CAD build for the part. Positions are in the model's coordinates, mm. Face numbers are marked on the shaded views. Give positions to 0.01 mm unless a question says otherwise; leave off trailing zeros. Order: outer loops, then holes, each group sorted by start corner. A loop starts at its lowest first (then second) coordinate and runs counter-clockwise, first axis right, second up. Notation, with made-up numbers: (85.25, -12) -> (115.25, -12) arc R21 ccw to (115.25, 25) -> close; hole circle Ø4 at (-10, 48.5). An arc over 180 degrees is marked (long way). Answer as CSV lines item,"result".
```python
from build123d import *

# Parameters (mm, degrees)
SKETCH_1_W           = 4.9
SKETCH_1_H           = 5.8
EXTRUDE_1_DEPTH      = 0.95
FILLET_1_R           = 0.2
CHAMFER_1_SIZE       = 0.2
EXTRUDE_2_DEPTH      = 0.05
EXTRUDE_2_DEPTH_BACK = 0.05
SKETCH_2_W           = 0.41
SKETCH_2_H           = 0.61
CHAMFER_2_SIZE       = 0.05
EXTRUDE_3_DEPTH      = 0.05
EXTRUDE_3_DEPTH_BACK = 0.05
SKETCH_3_W           = 4.15
SKETCH_3_H           = 3.85
SKETCH_3_W_2         = 0.41
SKETCH_3_H_2         = 0.15
SKETCH_3_W_3         = 0.375
SKETCH_3_H_3         = 0.41
SKETCH_3_W_4         = 0.15
CHAMFER_3_SIZE       = 0.05
SKETCH_4_R           = 0.15
CUT_EXTRUDE_1_DEPTH  = 0.01


with BuildPart() as part:
    # Эскиз1 → Бобышка-Вытянуть1 (new body)
    with BuildSketch(Plane(origin=(0, 0, 0), x_dir=(1, 0, 0), z_dir=(0, 1, 0))):
        Rectangle(SKETCH_1_W, SKETCH_1_H)
    extrude(amount=EXTRUDE_1_DEPTH)

    # Скругление1
    fillet_1_edges = [part.edges().sort_by_distance(p)[0] for p in [
        (2.45, 0.475, 2.9),
        (-2.45, 0.475, 2.9),
        (-2.45, 0.475, -2.9),
        (2.45, 0.475, -2.9),
    ]]
    fillet(fillet_1_edges, radius=FILLET_1_R)

    # Фаска1
    chamfer_1_edges = [part.edges().sort_by_distance(p)[0] for p in [
        (-2.45, 0.95, 0),
        (0, 0.95, -2.9),
        (2.45, 0.95, 0),
        (0, 0.95, 2.9),
        (2.391421356, 0.95, 2.841421356),
        (-2.391421356, 0.95, 2.841421356),
        (2.391421356, 0.95, -2.841421356),
        (-2.391421356, 0.95, -2.841421356),
    ]]
    chamfer(chamfer_1_edges, length=CHAMFER_1_SIZE)

    # Эскиз2 → Бобышка-Вытянуть2 (add, two sides: drawn at the far end of the back side and taken through both)
    with BuildSketch(Plane.XZ.offset(-EXTRUDE_2_DEPTH_BACK)):
        with Locations((0.635, -2.745)):
            Rectangle(SKETCH_2_W, SKETCH_2_H)
        with Locations((1.905, -2.745)):
            Rectangle(SKETCH_2_W, SKETCH_2_H)
        with Locations((-0.635, -2.745)):
            Rectangle(SKETCH_2_W, SKETCH_2_H)
        with Locations((-1.905, -2.745)):
            Rectangle(SKETCH_2_W, SKETCH_2_H)
    extrude(amount=EXTRUDE_2_DEPTH + EXTRUDE_2_DEPTH_BACK)

    # Фаска2
    chamfer_2_edges = [part.edges().sort_by_distance(p)[0] for p in [
        (-2.11, 0, -3.05),
        (-1.7, 0, -3.05),
        (1.7, 0, -3.05),
        (2.11, 0, -3.05),
        (0.43, 0, -3.05),
        (0.84, 0, -3.05),
        (-0.84, 0, -3.05),
        (-0.43, 0, -3.05),
    ]]
    chamfer(chamfer_2_edges, length=CHAMFER_2_SIZE)

    # Эскиз3 → Бобышка-Вытянуть3 (add, two sides: drawn at the far end of the back side and taken through both)
    with BuildSketch(Plane.XZ.offset(-EXTRUDE_3_DEPTH_BACK)):
        with Locations((0, 0.685)):
            Rectangle(SKETCH_3_W, SKETCH_3_H)
        with Locations((1.905, 2.975)):
            Rectangle(SKETCH_3_W_2, SKETCH_3_H_2)
        Polygon((1.7, 2.61), (2.075, 2.61), (2.11, 2.61), (2.11, 2.9), (1.7, 2.9), align=None)
        with Locations((-1.905, 2.975)):
            Rectangle(SKETCH_3_W_2, SKETCH_3_H_2)
        Polygon((-2.11, 2.61), (-2.075, 2.61), (-1.7, 2.61), (-1.7, 2.9), (-2.11, 2.9), align=None)
        with Locations((2.2625, -0.5)):
            Rectangle(SKETCH_3_W_3, SKETCH_3_H_3)
        with Locations((2.525, -0.5)):
            Rectangle(SKETCH_3_W_4, SKETCH_3_H_3)
        with Locations((-2.2625, -0.5)):
            Rectangle(SKETCH_3_W_3, SKETCH_3_H_3)
        with Locations((-2.525, -0.5)):
            Rectangle(SKETCH_3_W_4, SKETCH_3_H_3)
    extrude(amount=EXTRUDE_3_DEPTH + EXTRUDE_3_DEPTH_BACK)

    # Фаска3
    # the kernel refuses this chamfer: 0.05 mm, written as the material it adds along each edge
    with BuildSketch(Plane(origin=(-1.7, -0.05, 2.61), x_dir=(-0.02749587661058742, 0, 0.9996219169112966), z_dir=(0, 1, 0)), Plane(origin=(1.7, -0.05, 2.61), x_dir=(-0.9996219169112966, 0, -0.02749587661058718), z_dir=(0, 1, 0))) as chamfer_3_piece_1:
        Polygon((CHAMFER_3_SIZE * 0.999621916911, CHAMFER_3_SIZE * 0.0274958766106), (-CHAMFER_3_SIZE * 0.0274958766106, CHAMFER_3_SIZE * 0.999621916911), (0, 0), align=None)
    extrude(amount=0.178584149)
    # the kernel refuses this chamfer: 0.05 mm, written as the material it takes off along each edge
    with BuildSketch(Plane(origin=(-2.6, -0.178584149, -0.295), x_dir=(0.9996219169112966, 0, 0.02749587661058634), z_dir=(0, 1, 0)), Plane(origin=(2.6, -0.178584149, -0.705), x_dir=(-0.9996219169112965, 0, -0.027495876610591732), z_dir=(0, 1, 0)), Plane(origin=(2.6, -0.178584149, -0.295), x_dir=(0.02749587661058736, 0, -0.9996219169112966), z_dir=(0, 1, 0))) as chamfer_3_2_piece_1:
        Polygon((CHAMFER_3_SIZE * 0.999621916911, CHAMFER_3_SIZE * 0.0274958766106), (-CHAMFER_3_SIZE * 0.0274958766106, CHAMFER_3_SIZE * 0.999621916911), (0, 0), align=None)
    extrude(amount=0.357168299, mode=Mode.SUBTRACT)
    with BuildSketch(Plane(origin=(-2.11, -0.178584149, 2.61), x_dir=(-0.02749587661058742, 0, 0.9996219169112966), z_dir=(0, 1, 0))) as chamfer_3_2_piece_2_section:
        Polygon((CHAMFER_3_SIZE * 0.999621916911, CHAMFER_3_SIZE * 0.0274958766106), (-CHAMFER_3_SIZE * 0.0274958766106, CHAMFER_3_SIZE * 0.999621916911), (0, 0), align=None)
    chamfer_3_2_piece_2 = extrude(amount=0.178584149, mode=Mode.PRIVATE)
    chamfer_3_2_piece_2 = split(chamfer_3_2_piece_2, bisect_by=Plane(origin=(-2.075, -0.025, 2.627820513), z_dir=(-1, 0, 0)), keep=Keep.TOP, mode=Mode.PRIVATE)
    add(chamfer_3_2_piece_2, mode=Mode.SUBTRACT)
    with BuildSketch(Plane(origin=(-1.7, -0.178584149, 3.05), x_dir=(-0.9996219169112966, 0, 0.027495876610587302), z_dir=(0, 1, 0)), Plane(origin=(2.11, -0.178584149, 3.05), x_dir=(-0.9996219169112966, 0, 0.02749587661058742), z_dir=(0, 1, 0)), Plane(origin=(-2.6, -0.178584149, -0.705), x_dir=(0.9996219169112966, 0, -0.02749587661058742), z_dir=(0, 1, 0)), Plane(origin=(-2.11, -0.178584149, 3.05), x_dir=(-0.02749587661058742, 0, -0.9996219169112966), z_dir=(0, 1, 0)), Plane(origin=(1.7, -0.178584149, 3.05), x_dir=(-0.027495876610591732, 0, -0.9996219169112965), z_dir=(0, 1, 0))) as chamfer_3_2_piece_3:
        Polygon((CHAMFER_3_SIZE * 0.999621916911, -CHAMFER_3_SIZE * 0.0274958766106), (-CHAMFER_3_SIZE * 0.0274958766106, -CHAMFER_3_SIZE * 0.999621916911), (0, 0), align=None)
    extrude(amount=0.357168299, mode=Mode.SUBTRACT)
    with BuildSketch(Plane(origin=(2.11, -0.178584149, 2.61), x_dir=(0.02749587661058742, 0, 0.9996219169112966), z_dir=(0, 1, 0))) as chamfer_3_2_piece_4_section:
        Polygon((CHAMFER_3_SIZE * 0.999621916911, -CHAMFER_3_SIZE * 0.0274958766106), (-CHAMFER_3_SIZE * 0.0274958766106, -CHAMFER_3_SIZE * 0.999621916911), (0, 0), align=None)
    chamfer_3_2_piece_4 = extrude(amount=0.178584149, mode=Mode.PRIVATE)
    chamfer_3_2_piece_4 = split(chamfer_3_2_piece_4, bisect_by=Plane(origin=(2.075, -0.025, 2.627820513), z_dir=(1, 0, 0)), keep=Keep.TOP, mode=Mode.PRIVATE)
    add(chamfer_3_2_piece_4, mode=Mode.SUBTRACT)

    # Эскиз4 → Вырез-Вытянуть1 (cut)
    with BuildSketch(Plane(origin=(0, 0.95, 0), x_dir=(1, 0, 0), z_dir=(0, 1, 0))):
        with Locations(Location((1.85, 2.3, 0), (0, 0, 270))):
            Circle(SKETCH_4_R)
    extrude(amount=-CUT_EXTRUDE_1_DEPTH, mode=Mode.SUBTRACT)


solid = part.part
```
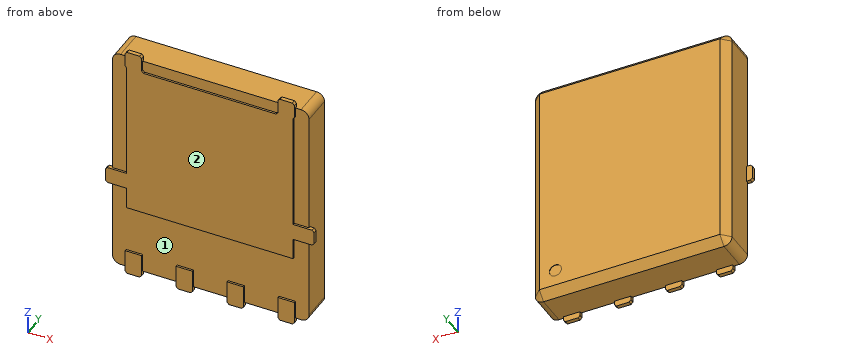
1) Pin check, flat tip, straight feed: P1, Ø0.6, axis at x = -0.5, y = 0.5, coming from the -Z side. Stop position of the tip, or through.
Data:
P1,"stops at z = -2.9"
2) Band-saw the part on A-A, the plane z = -1. Write the cut outline in (x, y) (3 decimals).
Data:
outline,"(-2.45, 0) -> (-2.075, 0) -> (-2.075, -0.05) -> (2.075, -0.05) -> (2.075, 0) -> (2.45, 0) -> (2.45, 0.75) -> (2.25, 0.95) -> (-2.25, 0.95) -> (-2.45, 0.75) -> close"
3) Wall check: line 1 along X through (y, z) = (0.3, 0); line 2 along Y through (x, z) = (2.2, 0.75); line 3 along Z through (x, y) = (0.7, 0.35). Give the ranges that are in metal, low to high. Write a range as [from, to].
Data:
line 1,"x = [-2.45, 2.45]"
line 2,"y = [0, 0.95]"
line 3,"z = [-2.9, 2.9]"
4) Pull direction X, two halves, no side cores. Call the marked faces 1 and 2: pulls with the +X half, pulls with the -X half, needs draft (parallel to the pull), parting line crosses it, or undercut.
Data:
face 1,"undercut"
face 2,"needs draft"
5) Band-saw the part on C-C, the plane y = 0.55. Write the cut outline in (x, z), then the cut area to 3 significant figures.
Data:
outline,"(-2.45, -2.7) arc R0.2 ccw to (-2.25, -2.9) -> (2.25, -2.9) arc R0.2 ccw to (2.45, -2.7) -> (2.45, 2.7) arc R0.2 ccw to (2.25, 2.9) -> (-2.25, 2.9) arc R0.2 ccw to (-2.45, 2.7) -> close"
area,"28.4 mm2"
